```python
from build123d import *

# Parameters (mm, degrees)
SKETCH1_R           = 4.1
BOSS_EXTRUDE1_DEPTH = 12.8
SKETCH2_R           = 2.75
CUT_EXTRUDE1_DEPTH  = 30.609218923


with BuildPart() as part:
    # Sketch1 → Boss-Extrude1 (new body)
    with BuildSketch(Plane.XY):
        with BuildLine():
            Line((-27.5, 4.5), (-27.5, 0))
            Line((-27.5, 0), (27.5, 0))
            Line((27.5, 0), (27.5, 4.5))
            Line((27.5, 4.5), (14.709218923, 4.5))
            Line((14.709218923, 4.5), (14.709218923, 14.9))
            ThreePointArc((14.709218923, 14.9), (0, 29.609218923), (-14.709218923, 14.9))
            Line((-14.709218923, 14.9), (-14.709218923, 4.5))
            Line((-14.709218923, 4.5), (-27.5, 4.5))
        make_face()
        with Locations((0, 14.9)):
            Circle(SKETCH1_R, mode=Mode.SUBTRACT)
    extrude(amount=BOSS_EXTRUDE1_DEPTH)

    # Sketch2 → Cut-Extrude1 (cut, through all)
    with BuildSketch(Plane.XZ):
        with Locations((-20.75, 6.4)):
            Circle(SKETCH2_R)
        with Locations((20.75, 6.4)):
            Circle(SKETCH2_R)
    extrude(amount=-CUT_EXTRUDE1_DEPTH, mode=Mode.SUBTRACT)


solid = part.part
```
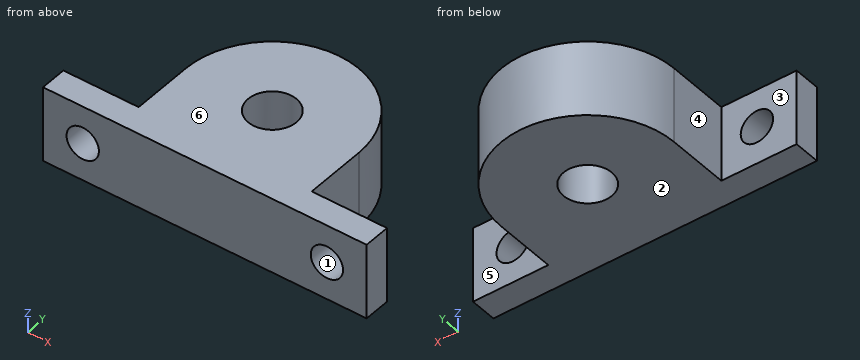
Model file for the job. Use its own axes, mm. Face numbers are marked on the shaded views. A direction names the side the tool comes from. Round coordinates to 2 decimals unless told otherwise and drop trailing zeros. Order: outer loops, then holes, each group sorted by start corner. A loop starts at its lowest first (then second) coordinate and runs counter-clockwise, first axis right, second up. Notation, with made-up numbers: (-29, 7.25) -> (12, 7.25) arc R18 ccw to (12, 30.25) -> close; hole circle Ø1 at (36, 80.5). An arc over 180 degrees is marked (long way). Use one line per item in the form item = value.
Item 1: Flat gauge pins, fed straight in: pin 1 Ø3 at (y, z) = (8, 4) entering from -X; pin 2 Ø2 at (y, z) = (15.5, 8) entering from +X; pin 3 Ø1.5 at (x, z) = (-12, 9) entering from +Y. Where does each tip first touch, or does it go through?
Returned:
pin_1 = -14.71
pin_2 = 14.71
pin_3 = 24.38
Item 2: Drill centre lines: line 1 (Z direction, x = -20.75, y = 3.25); line 2 (Y direction, x = 0, z = 9.5); line 3 (X direction, y = 15, z = 3.5). Where is each one in solid material? Low to high.
Returned:
line_1 = 0 to 3.65, 9.15 to 12.8
line_2 = 0 to 10.8, 19 to 29.61
line_3 = -14.71 to -4.1, 4.1 to 14.71
Item 3: Cut at D-D, the plane z = 10.5. Write the cut outline in (x, y), and give its area (4 significant figures).
Returned:
outline = (-27.5, 0) -> (27.5, 0) -> (27.5, 4.5) -> (14.71, 4.5) -> (14.71, 14.9) arc R14.71 ccw to (-14.71, 14.9) -> (-14.71, 4.5) -> (-27.5, 4.5) -> close; hole circle Ø8.2 at (0, 14.9)
area = 840.5 mm^2
Item 4: Pull direction Z, two halves, no side cores. Call the marked faces 1, 2 and 3: released by +Z, released by -Z, zero draft, split by the parting line, or undercut.
Returned:
face_1 = undercut
face_2 = released by -Z
face_3 = zero draft
Item 5: Cut at B-B, the plane x = 0. Write the cut outline in (y, z), and give its area (3 significant figures).
Returned:
outline = (0, 0) -> (10.8, 0) -> (10.8, 12.8) -> (0, 12.8) -> close; (19, 0) -> (29.61, 0) -> (29.61, 12.8) -> (19, 12.8) -> close
area = 274 mm^2
Item 6: Cut at A-A, the plane z = 6.4. Write the cut outline in (x, y).
Returned:
outline = (-27.5, 0) -> (-23.5, 0) -> (-23.5, 4.5) -> (-27.5, 4.5) -> close; (-18, 0) -> (18, 0) -> (18, 4.5) -> (14.71, 4.5) -> (14.71, 14.9) arc R14.71 ccw to (-14.71, 14.9) -> (-14.71, 4.5) -> (-18, 4.5) -> close; (23.5, 0) -> (27.5, 0) -> (27.5, 4.5) -> (23.5, 4.5) -> close; hole circle Ø8.2 at (0, 14.9)
Item 7: Cut at C-C, the plane y = 16.5. Write the cut outline in (x, z), and give its area (3 significant figures).
Returned:
outline = (-14.62, 0) -> (-3.77, 0) -> (-3.77, 12.8) -> (-14.62, 12.8) -> close; (3.77, 0) -> (14.62, 0) -> (14.62, 12.8) -> (3.77, 12.8) -> close
area = 278 mm^2
Item 8: Tool access for the marked faces 4, 5 and 6: list every direction of +Z, -Z, +X, -X, +Y, -Y with a clear straight run to the whole face (end or side of a thin tool).
Returned:
face_4 = +Z, -Z, -X, +Y
face_5 = +Z, -Z, +X, +Y
face_6 = +Z, +X, -X, +Y, -Y
